Geometry: final body of the model. Coordinates: model frame, mm. Face numbers are marked on the shaded views. A direction names the side the tool comes from. Give positions to 0.01 mm unless a question says otherwise; leave off trailing zeros. Loops run counter-clockwise (first coordinate to the right, second up) from the corner with the lowest first, then second, coordinate; pieces in that order, holes last. Notation, with made-up numbers: (-36.75, 23) - (-2.75, 23) arc R26 ccw to (-2.75, 44) - close; hole circle Ø11 at (-34.5, -11). An arc over 180 degrees is marked (long way). Answer in a Markdown table with one row per item.
from build123d import *

# Parameters (mm, degrees)
CROQUIS1_W                 = 62
CROQUIS1_H                 = 62
SALIENTE_EXTRUIR1_DEPTH    = 13
REDONDEO1_R                = 10
REDONDEO2_R                = 10
VACIADO1_T                 = -2.5
CROQUIS2_R                 = 21
CORTAR_EXTRUIR1_DEPTH      = 7
SALIENTE_EXTRUIR2_DEPTH    = 5
CROQUIS6_R                 = 12.25
CORTAR_EXTRUIR4_DEPTH      = 4
REDONDEO3_R                = 10
CROQUIS8_R                 = 3.813498279
SALIENTE_EXTRUIR3_DEPTH    = 13
REDONDEO4_R                = 3
CORTAR_EXTRUIR7_DEPTH      = 71.52659088
CORTAR_EXTRUIR7_DEPTH_BACK = 71.52659088
CROQUIS9_R                 = 1.65
CHAFL_N1_SIZE              = 1
CHAFL_N2_SIZE              = 1
CHAFL_N3_SIZE              = 1
CHAFL_N4_SIZE              = 0.4
CHAFL_N4_SIZE2             = 1.098990968
CHAFL_N5_SIZE              = 1
CROQUIS10_R                = 14.000593708
CROQUIS10_R_2              = 10.396987038
SALIENTE_EXTRUIR4_DEPTH    = 0.5
CROQUIS11_R                = 9.192870702
CORTAR_EXTRUIR8_DEPTH      = 71.349129497
CHAFL_N6_SIZE              = 0.75


with BuildPart() as part:
    # Croquis1 → Saliente-Extruir1 (new body)
    with BuildSketch(Plane(origin=(0, 0, 0), x_dir=(1, 0, 0), z_dir=(0, 1, 0))):
        with Locations((31, 0)):
            Rectangle(CROQUIS1_W, CROQUIS1_H)
    extrude(amount=SALIENTE_EXTRUIR1_DEPTH)

    # Redondeo1
    redondeo1_edges = [part.edges().sort_by_distance(p)[0] for p in [
        (62, 6.5, -31),
        (62, 6.5, 31),
    ]]
    fillet(redondeo1_edges, radius=REDONDEO1_R)

    # Redondeo2
    redondeo2_edges = [part.edges().sort_by_distance(p)[0] for p in [
        (0, 6.5, -31),
        (0, 6.5, 31),
    ]]
    fillet(redondeo2_edges, radius=REDONDEO2_R)

    # Vaciado1
    vaciado1_openings = [part.faces().sort_by_distance(p)[0] for p in [
        (31, 13, 0),
        (31, 0, 0),
    ]]
    offset(amount=VACIADO1_T, openings=vaciado1_openings, kind=Kind.INTERSECTION)

    # Croquis2 → Cortar-Extruir1 (cut)
    with BuildSketch(Plane(origin=(0, 13, 0), x_dir=(1, 0, 0), z_dir=(0, 1, 0))):
        with Locations((16.5, 0)):
            Circle(CROQUIS2_R)
    extrude(amount=-CORTAR_EXTRUIR1_DEPTH, mode=Mode.SUBTRACT)

    # Croquis4 → Saliente-Extruir2 (add)
    with BuildSketch(Plane.XZ):
        with BuildLine():
            Line((7.085748882, 29.157404391), (31.085748882, 29.157404391))
            Line((31.085748882, 29.157404391), (31.085748882, -29.960159471))
            Line((31.085748882, -29.960159471), (7.085748882, -29.960159471))
            ThreePointArc((7.085748882, -29.960159471), (3.550214976, -28.495693377), (2.085748882, -24.960159471))
            Line((2.085748882, -24.960159471), (2.085748882, 24.157404391))
            ThreePointArc((2.085748882, 24.157404391), (3.550214976, 27.692938297), (7.085748882, 29.157404391))
        make_face()
    extrude(amount=-SALIENTE_EXTRUIR2_DEPTH)

    # Croquis6 → Cortar-Extruir4 (cut)
    with BuildSketch(Plane(origin=(0, 5, 0), x_dir=(1, 0, 0), z_dir=(0, 1, 0))):
        with Locations(Location((16.5, 0, 0), (0, 0, 270))):
            Circle(CROQUIS6_R)
    extrude(amount=-CORTAR_EXTRUIR4_DEPTH, mode=Mode.SUBTRACT)

    # Redondeo3
    redondeo3_edges = [part.edges().sort_by_distance(p)[0] for p in [
        (31.085748882, 2.5, -28.5),
        (31.085748882, 2.5, 28.5),
    ]]
    fillet(redondeo3_edges, radius=REDONDEO3_R)

    # Croquis8 → Saliente-Extruir3 (add)
    with BuildSketch(Plane(origin=(0, 13, 0), x_dir=(1, 0, 0), z_dir=(0, 1, 0))):
        with Locations((55.43014903, 24.042715564)):
            Circle(CROQUIS8_R)
        with Locations((55.43014903, -24.042715564)):
            Circle(CROQUIS8_R)
    extrude(amount=-SALIENTE_EXTRUIR3_DEPTH)

    # Redondeo4
    redondeo4_edges = [part.edges().sort_by_distance(p)[0] for p in [
        (55.076843568, 6.5, 27.839812399),
        (59.157992619, 6.5, 23.239004614),
        (59.157992619, 6.5, -23.239004614),
        (55.076843568, 6.5, -27.839812399),
    ]]
    fillet(redondeo4_edges, radius=REDONDEO4_R)

    # Croquis9 → Cortar-Extruir7 (cut, two sides: drawn at the far end of the back side and taken through both)
    with BuildSketch(Plane(origin=(0, 13, 0), x_dir=(1, 0, 0), z_dir=(0, 1, 0)).offset(-CORTAR_EXTRUIR7_DEPTH_BACK)):
        with Locations(Location((6, 25, 0), (0, 0, 270))):
            Circle(CROQUIS9_R)
        with Locations(Location((56, -25, 0), (0, 0, 270))):
            Circle(CROQUIS9_R)
        with Locations(Location((56, 25, 0), (0, 0, 270))):
            Circle(CROQUIS9_R)
        with Locations(Location((6, -25, 0), (0, 0, 270))):
            Circle(CROQUIS9_R)
    extrude(amount=CORTAR_EXTRUIR7_DEPTH + CORTAR_EXTRUIR7_DEPTH_BACK, mode=Mode.SUBTRACT)

    # Chaflán1
    # the kernel refuses this chamfer: 1 mm, written as the material it takes off along each edge
    with BuildSketch(Plane(origin=(6, 5, 25), x_dir=(0, 0, 1), z_dir=(-1, 0, 0))) as chafl_n1_piece_1_section:
        Polygon((1.65, -CHAFL_N1_SIZE), (1.65 + CHAFL_N1_SIZE, 0), (1.65, 0), align=None)
    chafl_n1_piece_1 = revolve(axis=Axis((6, 5, 25), (0, 1, 0)), mode=Mode.PRIVATE)
    chafl_n1_piece_1 = chafl_n1_piece_1 & Plane(origin=(10, 4.51284456, 21), x_dir=(-1, 0, 0), z_dir=(0, 1, 0)) * Cylinder(7.5, 11, mode=Mode.PRIVATE)
    add(chafl_n1_piece_1, mode=Mode.SUBTRACT)
    with BuildSketch(Plane(origin=(56, 13, -25), x_dir=(0, 0, 1), z_dir=(-1, 0, 0))) as chafl_n1_piece_2:
        Polygon((1.65, -CHAFL_N1_SIZE), (1.65 + CHAFL_N1_SIZE, 0), (1.65, 0), align=None)
    revolve(axis=Axis((56, 13, -25), (0, 1, 0)), mode=Mode.SUBTRACT)
    with BuildSketch(Plane(origin=(56, 13, 25), x_dir=(0, 0, 1), z_dir=(-1, 0, 0))) as chafl_n1_piece_3:
        Polygon((1.65, -CHAFL_N1_SIZE), (1.65 + CHAFL_N1_SIZE, 0), (1.65, 0), align=None)
    revolve(axis=Axis((56, 13, 25), (0, 1, 0)), mode=Mode.SUBTRACT)
    with BuildSketch(Plane(origin=(6, 5, -25), x_dir=(0, 0, 1), z_dir=(-1, 0, 0))) as chafl_n1_piece_4_section:
        Polygon((1.65, -CHAFL_N1_SIZE), (1.65 + CHAFL_N1_SIZE, 0), (1.65, 0), align=None)
    chafl_n1_piece_4 = revolve(axis=Axis((6, 5, -25), (0, 1, 0)), mode=Mode.PRIVATE)
    chafl_n1_piece_4 = chafl_n1_piece_4 & Plane(origin=(10, 4.512844583, -21), x_dir=(0, 0, -1), z_dir=(0, 1, 0)) * Cylinder(7.5, 11, mode=Mode.PRIVATE)
    add(chafl_n1_piece_4, mode=Mode.SUBTRACT)

    # Chaflán2
    chafl_n2_edges = [part.edges().sort_by_distance(p)[0] for p in [
        (16.5, 5, -12.25),
    ]]
    chamfer(chafl_n2_edges, length=CHAFL_N2_SIZE)

    # Chaflán3
    chafl_n3_edges = [part.edges().sort_by_distance(p)[0] for p in [
        (31.085748882, 5, 0),
        (34.01468107, 5, 25.571067812),
        (34.01468107, 5, -25.571067812),
    ]]
    chamfer(chafl_n3_edges, length=CHAFL_N3_SIZE)

    # Chaflán4
    chafl_n4_edges = [part.edges().sort_by_distance(p)[0] for p in [
        (31, 0, -31),
        (62, 0, 0),
        (59.071067812, 0, 28.071067812),
        (59.071067812, 0, -28.071067812),
        (31, 0, 31),
        (0, 0, 0),
        (2.928932188, 0, -28.071067812),
        (2.928932188, 0, 28.071067812),
    ]]
    chafl_n4_side = [part.faces().sort_by_distance(p)[0] for p in [
        (22.290109536, 0, 0),
    ]]
    chamfer(chafl_n4_edges, length=CHAFL_N4_SIZE, length2=CHAFL_N4_SIZE2, reference=chafl_n4_side[0])

    # Chaflán5
    chafl_n5_edges = [part.edges().sort_by_distance(p)[0] for p in [
        (6, 0, 23.35),
        (56, 0, -26.65),
        (56, 0, 23.35),
        (6, 0, -26.65),
    ]]
    chamfer(chafl_n5_edges, length=CHAFL_N5_SIZE)

    # Croquis10 → Saliente-Extruir4 (add)
    with BuildSketch(Plane(origin=(0, 1, 0), x_dir=(1, 0, 0), z_dir=(0, 1, 0))):
        with Locations((16.5, 0)):
            Circle(CROQUIS10_R)
        with Locations(Location((16.5, 0, 0), (0, 0, 270))):
            Circle(CROQUIS10_R_2, mode=Mode.SUBTRACT)
    extrude(amount=SALIENTE_EXTRUIR4_DEPTH)

    # Croquis11 → Cortar-Extruir8 (cut, through all)
    with BuildSketch(Plane(origin=(0, 1, 0), x_dir=(1, 0, 0), z_dir=(0, 1, 0))):
        with Locations(Location((16.5, 0, 0), (0, 0, 270))):
            Circle(CROQUIS11_R)
    extrude(amount=-CORTAR_EXTRUIR8_DEPTH, mode=Mode.SUBTRACT)

    # Chaflán6
    chafl_n6_edges = [part.edges().sort_by_distance(p)[0] for p in [
        (8.173443839, 5, 28.274179857),
        (23.251586594, 5, 28.5),
        (8.173443839, 5, -28.274179857),
        (23.251586594, 5, -28.5),
    ]]
    chamfer(chafl_n6_edges, length=CHAFL_N6_SIZE)


solid = part.part
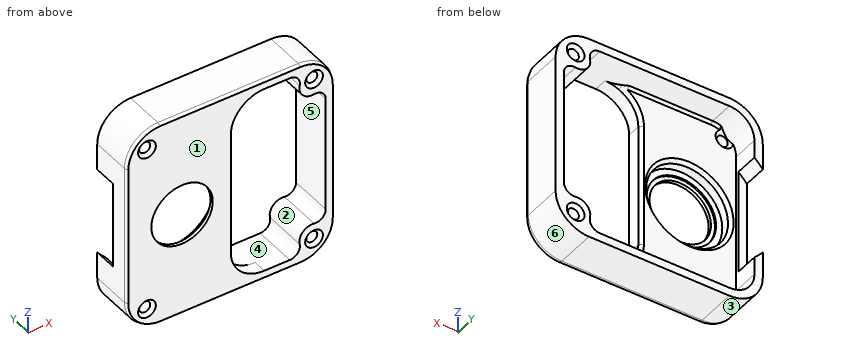
Q1. Draft query along Z for the marked faces 1, 2 and 3. Return one class per face: pulls with the +Z half, pulls with the -Z half, needs draft (parallel to the pull), parting line crosses it, or undercut.
Check values:
| item | result |
|---|---|
| face 1 | needs draft |
| face 2 | undercut |
| face 3 | pulls with the -Z half |
Q2. Cut plane D-D (x = 44). Output: boundary loops of the cut face in (y, z), and give its area (3 significant figures).
Check values:
| item | result |
|---|---|
| outline | (0, -30.6) - (1.1, -31) - (13, -31) - (13, -28.5) - (0, -28.5) - close; (0, 28.5) - (13, 28.5) - (13, 31) - (1.1, 31) - (0, 30.6) - close |
| area | 64.6 mm² |
Q3. Cut plane A-A (x = 16.5). Output: boundary loops of the cut face in (y, z), and give its area (3 significant figures).
Check values:
| item | result |
|---|---|
| outline | (0, -30.6) - (1.1, -31) - (13, -31) - (13, -28.5) - (5.75, -28.5) - (5, -27.75) - (5, -13.25) - (4, -12.25) - (1.5, -12.25) - (1.5, -10.4) - (1, -10.4) - (1, -9.19) - (0, -9.19) - close; (0, 9.19) - (1, 9.19) - (1, 10.4) - (1.5, 10.4) - (1.5, 12.25) - (4, 12.25) - (5, 13.25) - (5, 27.75) - (5.75, 28.5) - (13, 28.5) - (13, 31) - (1.1, 31) - (0, 30.6) - close |
| area | 235 mm² |
Q4. Cut plane B-B (z = 0). Output: boundary loops of the cut face in (x, y), and give its area (3 significant figures).
Check values:
| item | result |
|---|---|
| outline | (0, 1.1) - (0.4, 0) - (7.31, 0) - (7.31, 1) - (6.1, 1) - (6.1, 1.5) - (4.25, 1.5) - (4.25, 4) - (3.25, 5) - (2.5, 5) - (2.5, 6) - (0, 6) - close; (25.69, 0) - (31.09, 0) - (31.09, 4) - (30.09, 5) - (29.75, 5) - (28.75, 4) - (28.75, 1.5) - (26.9, 1.5) - (26.9, 1) - (25.69, 1) - close; (59.5, 0) - (61.6, 0) - (62, 1.1) - (62, 13) - (59.5, 13) - close |
| area | 74.0 mm² |
Q5. Reachability of the marked faces 4, 5 and 6 from +Z, -Z, +X, -X, +Y, -Y: full face, straight path, thin tool, end or side. Return the list, or none.
Check values:
| item | result |
|---|---|
| face 4 | +Y |
| face 5 | +Y, -Y |
| face 6 | -Z, +X, +Y, -Y |
Q6. Material intervals for line 1 along X through (y, z) = (1.1, 0); line 2 along Z through (x, y) = (15.5, 6.5); line 3 along Z through (x, y) = (56, 8.75), sorted ascending.
Check values:
| item | result |
|---|---|
| line 1 | 0 to 6.1, 26.9 to 31.09, 59.5 to 62 |
| line 2 | -31 to -28.5, 28.5 to 31 |
| line 3 | -30.17 to -26.65, -23.35 to -20.27, 20.27 to 23.35, 26.65 to 30.17 |
Q7. First-contact query: pin 1 (2 mm diameter, centred on x = 56, z = 25, fed in from -Y); pin 2 (5 mm diameter, centred on x = 6.5, z = -2.5, fed in from +Y); pin 3 (4 mm diameter, centred on x = 6, z = -25, fed in from -Y); pin 4 (23 mm diameter, centred on x = 20.5, z = 4, fed in from +Y). Flat tips, straight axial feed; report the tip coordinate or a pass-through.
Check values:
| item | result |
|---|---|
| pin 1 | through |
| pin 2 | y = 4.56 |
| pin 3 | y = 0.65 |
| pin 4 | y = 5 |
Q8. Cut plane C-C (z = -14). Output: boundary loops of the cut face in (x, y), and give its area (3 significant figures).
Check values:
| item | result |
|---|---|
| outline | (0, 1.1) - (0.4, 0) - (31.09, 0) - (31.09, 4) - (30.09, 5) - (2.5, 5) - (2.5, 6) - (0.85, 6) - (0.85, 13) - (0, 13) - close; (59.5, 0) - (61.6, 0) - (62, 1.1) - (62, 13) - (59.5, 13) - close |
| area | 195 mm² |
